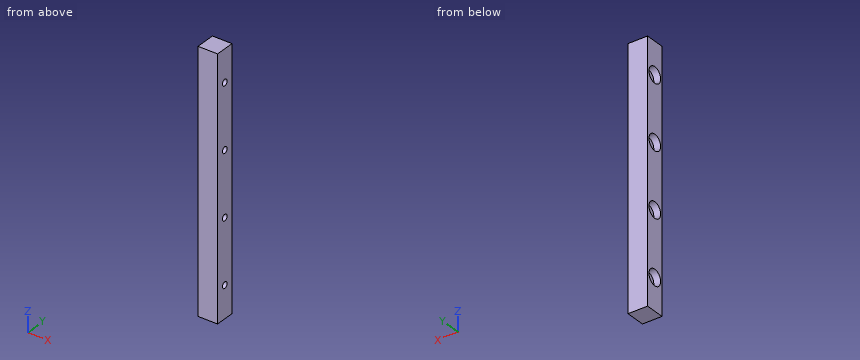
from build123d import *

# Parameters (mm, degrees)
SKETCH1_W           = 13
SKETCH1_H           = 13
BOSS_EXTRUDE1_DEPTH = 85
SKETCH2_R           = 2.1
CUT_EXTRUDE1_DEPTH  = 11.5
SKETCH3_R           = 5.25
CUT_EXTRUDE2_DEPTH  = 4.5


with BuildPart() as part:
    # Sketch1 → Boss-Extrude1 (new, symmetric)
    with BuildSketch(Plane.XY):
        Rectangle(SKETCH1_W, SKETCH1_H)
    extrude(amount=BOSS_EXTRUDE1_DEPTH, both=True)

    # Sketch2 → Cut-Extrude1 (cut, symmetric)
    with BuildSketch(Plane(origin=(0, 0, 0), x_dir=(0, 0, -1), z_dir=(1, 0, 0))):
        with Locations((63.75, 0)):
            Circle(SKETCH2_R)
        with Locations((21.25, 0)):
            Circle(SKETCH2_R)
        with Locations((-21.25, 0)):
            Circle(SKETCH2_R)
        with Locations((-63.75, 0)):
            Circle(SKETCH2_R)
    extrude(amount=CUT_EXTRUDE1_DEPTH, both=True, mode=Mode.SUBTRACT)

    # Sketch3 → Cut-Extrude2 (cut, symmetric)
    with BuildSketch(Plane(origin=(-6.5, 0, 0), x_dir=(0, 0, -1), z_dir=(1, 0, 0))):
        with Locations((63.75, 0)):
            Circle(SKETCH3_R)
        with Locations((21.25, 0)):
            Circle(SKETCH3_R)
        with Locations((-21.25, 0)):
            Circle(SKETCH3_R)
        with Locations((-63.75, 0)):
            Circle(SKETCH3_R)
    extrude(amount=CUT_EXTRUDE2_DEPTH, both=True, mode=Mode.SUBTRACT)


solid = part.part
The listing builds one solid part. Answer for the finished solid, in the listing's coordinates (mm). Give positions to 0.01 mm unless a question says otherwise; leave off trailing zeros. Write each loop counter-clockwise with the first axis right and the second up, starting at its lowest first coordinate (ties: lowest second). Pieces come first, ordered by that corner, then holes. Notation, with made-up numbers: (-24, -18.5) -> (6, -18.5) arc R19 cw to (6, -2.5) -> close; hole circle Ø8 at (34, 41). An arc over 180 degrees is marked (long way). One line per question, with ' | ' between items. Start each with the question number.
1. Section A-A (x = 2) is taken. Determine the outline of the cut face in (y, z).
2. Section B-B (z = 63.75) is taken. Determine the outline of the cut face in (x, y).
3. Given pin 1 Ø4 at (y, z) = (0, -63.75) entering from -X; pin 2 Ø5 at (y, z) = (0, 21.25) entering from -X, each flat-ended and moving along its own axis, determine where each tip first touches the part or whether it passes through.
4. Section C-C (x = -4) is taken. Determine the outline of the cut face in (y, z), plus the area to 3 significant figures.
5. Find the intervals of material crossed by probe 1 along Y at (x, z) = (-3, -21.25); probe 2 along Z at (x, y) = (2, 1.5); probe 3 along Y at (x, z) = (4.75, -21.25), in increasing order.
Response values:
1) outline: (-6.5, -85) -> (6.5, -85) -> (6.5, 85) -> (-6.5, 85) -> close; hole circle Ø4.2 at (0, -63.75); hole circle Ø4.2 at (0, -21.25); hole circle Ø4.2 at (0, 21.25); hole circle Ø4.2 at (0, 63.75)
2) outline: (-6.5, -6.5) -> (6.5, -6.5) -> (6.5, -2.1) -> (-2, -2.1) -> (-2, -5.25) -> (-6.5, -5.25) -> close; (-6.5, 5.25) -> (-2, 5.25) -> (-2, 2.1) -> (6.5, 2.1) -> (6.5, 6.5) -> (-6.5, 6.5) -> close
3) pin 1: through | pin 2: x = -2
4) outline: (-6.5, -85) -> (6.5, -85) -> (6.5, 85) -> (-6.5, 85) -> close; hole circle Ø10.5 at (0, -63.75); hole circle Ø10.5 at (0, -21.25); hole circle Ø10.5 at (0, 21.25); hole circle Ø10.5 at (0, 63.75) | area: 1,860 mm2
5) probe 1: -6.5 to -5.25, 5.25 to 6.5 | probe 2: -85 to -65.22, -62.28 to -22.72, -19.78 to 19.78, 22.72 to 62.28, 65.22 to 85 | probe 3: -6.5 to -2.1, 2.1 to 6.5
